For this review, take the finished solid that the model builds, in its own axes (mm). A direction names the side the tool comes from. Give positions to 0.01 mm unless a question says otherwise; leave off trailing zeros. Loops run counter-clockwise (first coordinate to the right, second up) from the corner with the lowest first, then second, coordinate; pieces in that order, holes last.
```python
from build123d import *

# Parameters (mm, degrees)
SKETCH1_R           = 19.05
BOSS_EXTRUDE1_DEPTH = 101.6
SKETCH2_R           = 15.875
CUT_EXTRUDE1_DEPTH  = 101.6
SKETCH3_R           = 25.4
BOSS_EXTRUDE2_DEPTH = 12.7
SKETCH4_R           = 15.875
CUT_EXTRUDE2_DEPTH  = 12.7


with BuildPart() as part:
    # Sketch1 → Boss-Extrude1 (new body)
    with BuildSketch(Plane.XY):
        Circle(SKETCH1_R)
    extrude(amount=BOSS_EXTRUDE1_DEPTH)

    # Sketch2 → Cut-Extrude1 (cut)
    with BuildSketch(Plane.XY.offset(101.6)):
        Circle(SKETCH2_R)
    extrude(amount=-CUT_EXTRUDE1_DEPTH, mode=Mode.SUBTRACT)

    # Sketch3 → Boss-Extrude2 (add)
    with BuildSketch(Plane.XY.offset(101.6)):
        Circle(SKETCH3_R)
    extrude(amount=-BOSS_EXTRUDE2_DEPTH)

    # Sketch4 → Cut-Extrude2 (cut)
    with BuildSketch(Plane.XY.offset(101.6)):
        Circle(SKETCH4_R)
    extrude(amount=-CUT_EXTRUDE2_DEPTH, mode=Mode.SUBTRACT)


solid = part.part
```
Q1. Machinability: for faces 4 (the flat face through (4, 19, 88.9)), 5 (the flat face through (-4, 16, 0)), which of the approach directions +Z, -Z, +X, -X, +Y, -Y give a long, thin tool a straight path to every point of the face, cutting with its end or side? Answer none if there is none.
Answers:
face 4: -Z
face 5: -Z, +X, -X, +Y, -Y
Q2. For probe 1 along Y at (x, z) = (0, 50.5) (3 decimals); probe 2 along X at (y, z) = (8, 43); probe 3 along Z at (x, y) = (-8, 19.5), list the stretches that pass through material, from the lowest coordinate up.
Answers:
probe 1: y = -19.05 to -15.875, 15.875 to 19.05
probe 2: x = -17.29 to -13.71, 13.71 to 17.29
probe 3: z = 88.9 to 101.6
Q3. Consider section A-A on y = 0. Give the boundary of the cut face in (x, z) (3 decimals).
Answers:
outline: (-25.4, 88.9) - (-19.05, 88.9) - (-19.05, 0) - (-15.875, 0) - (-15.875, 101.6) - (-25.4, 101.6) - close; (15.875, 0) - (19.05, 0) - (19.05, 88.9) - (25.4, 88.9) - (25.4, 101.6) - (15.875, 101.6) - close
Q4. Consider section D-D on x = -17. Give the boundary of the cut face in (y, z).
Answers:
outline: (-18.87, 88.9) - (-8.6, 88.9) - (-8.6, 0) - (8.6, 0) - (8.6, 88.9) - (18.87, 88.9) - (18.87, 101.6) - (-18.87, 101.6) - close
Q5. For pin 1 Ø2 at (x, z) = (4, 78) entering from -Y; pin 2 Ø2 at (x, z) = (-4.5, 79) entering from +Y; pin 3 Ø8 at (y, z) = (10, 30.5) entering from +X, all flat-tipped, find the tip position at first contact; note any pin that passes through.
Answers:
pin 1: stops at y = -18.81
pin 2: stops at y = 18.73
pin 3: stops at x = 18.08
Q6. Consider section C-C on z = 15. Give the boundary of the cut face in (x, y) (3 decimals), plus the area to 3 significant figures.
Answers:
outline: circle Ø38.1 at (0, 0); hole circle Ø31.75 at (0, 0)
area: 348 mm2
Q7. Mouldability with a two-part tool opening along Y and no side actions: class faces 1 (the cylindrical face through (-3.441, -15.497, 51.511)), 2 (the cylindrical face through (-5.506, -24.796, 95.339)), 3 (the flat face through (11, 12, 101.6)) as +Y half, -Y half, draft (parallel to the pull), parting line (faces both ways), or undercut.
Answers:
face 1: undercut
face 2: parting line
face 3: draft
